```python
from build123d import *

# Parameters (mm, degrees)
BOSS_EXTRUDE1_DEPTH = 25
FILLET1_R           = 5
SKETCH2_R           = 2
CUT_EXTRUDE1_DEPTH  = 5
FILLET2_R           = 5
BOSS_EXTRUDE2_DEPTH = 2.5
FILLET3_R           = 5
FILLET4_R           = 3


with BuildPart() as part:
    # Sketch1 → Boss-Extrude1 (new, symmetric)
    with BuildSketch(Plane(origin=(0, 0, 0), x_dir=(1, 0, 0), z_dir=(0, 1, 0))):
        Polygon((-40, 0), (-20, 0), (-20, 40), (20, 40), (20, 0), (40, 0), (40, 5), (25, 5), (25, 45), (-25, 45), (-25, 5), (-40, 5), align=None)
    extrude(amount=BOSS_EXTRUDE1_DEPTH, both=True)

    # Fillet1
    fillet1_edges = [part.edges().sort_by_distance(p)[0] for p in [
        (-25, 0, -5),
        (-25, 0, -45),
        (25, 0, -45),
        (25, 0, -5),
        (20, 0, -40),
        (-20, 0, -40),
    ]]
    fillet(fillet1_edges, radius=FILLET1_R)

    # Sketch2 → Cut-Extrude1 (cut)
    with BuildSketch(Plane.XY):
        with Locations((-32.5, 20)):
            Circle(SKETCH2_R)
        with Locations((-32.5, -20)):
            Circle(SKETCH2_R)
        with Locations((32.5, -20)):
            Circle(SKETCH2_R)
        with Locations((32.5, 20)):
            Circle(SKETCH2_R)
    extrude(amount=-CUT_EXTRUDE1_DEPTH, mode=Mode.SUBTRACT)

    # Fillet2
    fillet2_edges = [part.edges().sort_by_distance(p)[0] for p in [
        (40, -25, -2.5),
        (-40, -25, -2.5),
        (40, 25, -2.5),
        (-40, 25, -2.5),
    ]]
    fillet(fillet2_edges, radius=FILLET2_R)

    # Sketch3 → Boss-Extrude2 (add, symmetric)
    with BuildSketch(Plane(origin=(0, 0, 0), x_dir=(1, 0, 0), z_dir=(0, 1, 0))):
        Polygon((-40, 5), (-25, 35), (-25, 5), align=None)
    boss_extrude2 = extrude(amount=BOSS_EXTRUDE2_DEPTH, both=True)

    # Mirror5: Boss-Extrude2 across plane
    add(boss_extrude2.mirror(Plane(origin=(0, 0, 0), x_dir=(0, 0, 1), z_dir=(1, 0, 0))))

    # Fillet3
    # the kernel refuses this fillet: 5 mm, written as the material it adds along each edge
    with BuildSketch(Plane(origin=(-30, -2.5, -10), x_dir=(1, 0, 0), z_dir=(0, 0, -1))) as fillet3_piece_1:
        with BuildLine():
            CenterArc((5 - FILLET3_R, FILLET3_R), FILLET3_R, 270, 90)
            Line((5 - FILLET3_R, 0), (5, 0))
            Line((5, 0), (5, FILLET3_R))
        make_face()
    revolve(axis=Axis((-30, -2.5, -10), (0, -1, 0)), revolution_arc=90)
    with BuildSketch(Plane(origin=(-30, 2.5, -10), x_dir=(1, 0, 0), z_dir=(0, 0, -1))) as fillet3_piece_2:
        with BuildLine():
            CenterArc((5 - FILLET3_R, -FILLET3_R), FILLET3_R, 0, 90)
            Line((5 - FILLET3_R, 0), (5, 0))
            Line((5, 0), (5, -FILLET3_R))
        make_face()
    revolve(axis=Axis((-30, 2.5, -10), (0, -1, 0)), revolution_arc=90)
    with BuildSketch(Plane(origin=(-25, -2.5, -47.5), x_dir=(-1, 0, 0), z_dir=(0, 0, 1))) as fillet3_piece_3_section:
        with BuildLine():
            CenterArc((FILLET3_R, FILLET3_R), FILLET3_R, 180, 90)
            Line((0, FILLET3_R), (0, 0))
            Line((0, 0), (FILLET3_R, 0))
        make_face()
    fillet3_piece_3 = extrude(amount=37.5, mode=Mode.PRIVATE)
    fillet3_piece_3 = split(fillet3_piece_3, bisect_by=Plane(origin=(-30.617859864, -3.692357018, -23.764280273), z_dir=(0.894427190999916, 0, 0.44721359549995787)), keep=Keep.TOP, mode=Mode.PRIVATE)
    add(fillet3_piece_3)
    with BuildSketch(Plane(origin=(-25, 2.5, -47.5), x_dir=(0, 1, 0), z_dir=(0, 0, 1))) as fillet3_piece_4_section:
        with BuildLine():
            CenterArc((FILLET3_R, FILLET3_R), FILLET3_R, 180, 90)
            Line((0, FILLET3_R), (0, 0))
            Line((0, 0), (FILLET3_R, 0))
        make_face()
    fillet3_piece_4 = extrude(amount=37.5, mode=Mode.PRIVATE)
    fillet3_piece_4 = split(fillet3_piece_4, bisect_by=Plane(origin=(-30.617859864, 3.692357018, -23.764280273), z_dir=(0.894427190999916, 0, 0.44721359549995787)), keep=Keep.TOP, mode=Mode.PRIVATE)
    add(fillet3_piece_4)
    with BuildSketch(Plane(origin=(-30, 2.5, -5), x_dir=(0, 1, 0), z_dir=(-1, 0, 0))) as fillet3_piece_5_section:
        with BuildLine():
            CenterArc((FILLET3_R, FILLET3_R), FILLET3_R, 180, 90)
            Line((0, FILLET3_R), (0, 0))
            Line((0, 0), (FILLET3_R, 0))
        make_face()
    fillet3_piece_5 = extrude(amount=10, mode=Mode.PRIVATE)
    fillet3_piece_5 = split(fillet3_piece_5, bisect_by=Plane(origin=(-38.518002001, 3.668083757, -7.963995998), z_dir=(0.894427190999916, 0, 0.44721359549995787)), keep=Keep.TOP, mode=Mode.PRIVATE)
    add(fillet3_piece_5)
    with BuildSketch(Plane(origin=(-30, -2.5, -5), x_dir=(0, -1, 0), z_dir=(-1, 0, 0))) as fillet3_piece_6_section:
        with BuildLine():
            CenterArc((FILLET3_R, -FILLET3_R), FILLET3_R, 90, 90)
            Line((0, -FILLET3_R), (0, 0))
            Line((0, 0), (FILLET3_R, 0))
        make_face()
    fillet3_piece_6 = extrude(amount=10, mode=Mode.PRIVATE)
    fillet3_piece_6 = split(fillet3_piece_6, bisect_by=Plane(origin=(-38.518002001, -3.668083757, -7.963995998), z_dir=(0.894427190999916, 0, 0.44721359549995787)), keep=Keep.TOP, mode=Mode.PRIVATE)
    add(fillet3_piece_6)
    with BuildSketch(Plane(origin=(30, -2.5, -10), x_dir=(-1, 0, 0), z_dir=(0, 0, -1))) as fillet3_piece_7:
        with BuildLine():
            CenterArc((5 - FILLET3_R, -FILLET3_R), FILLET3_R, 0, 90)
            Line((5 - FILLET3_R, 0), (5, 0))
            Line((5, 0), (5, -FILLET3_R))
        make_face()
    revolve(axis=Axis((30, -2.5, -10), (0, 1, 0)), revolution_arc=90)
    with BuildSketch(Plane(origin=(30, 2.5, -10), x_dir=(-1, 0, 0), z_dir=(0, 0, -1))) as fillet3_piece_8:
        with BuildLine():
            CenterArc((5 - FILLET3_R, FILLET3_R), FILLET3_R, 270, 90)
            Line((5, FILLET3_R), (5, 0))
            Line((5, 0), (5 - FILLET3_R, 0))
        make_face()
    revolve(axis=Axis((30, 2.5, -10), (0, 1, 0)), revolution_arc=90)
    with BuildSketch(Plane(origin=(25, 2.5, -47.5), x_dir=(0, 1, 0), z_dir=(0, 0, 1))) as fillet3_piece_9_section:
        with BuildLine():
            CenterArc((FILLET3_R, -FILLET3_R), FILLET3_R, 90, 90)
            Line((0, -FILLET3_R), (0, 0))
            Line((0, 0), (FILLET3_R, 0))
        make_face()
    fillet3_piece_9 = extrude(amount=37.5, mode=Mode.PRIVATE)
    fillet3_piece_9 = split(fillet3_piece_9, bisect_by=Plane(origin=(30.617859864, 3.692357018, -23.764280273), z_dir=(-0.894427190999916, 0, 0.44721359549995787)), keep=Keep.TOP, mode=Mode.PRIVATE)
    add(fillet3_piece_9)
    with BuildSketch(Plane(origin=(30, -2.5, -5), x_dir=(0, -1, 0), z_dir=(1, 0, 0))) as fillet3_piece_10_section:
        with BuildLine():
            CenterArc((FILLET3_R, FILLET3_R), FILLET3_R, 180, 90)
            Line((0, FILLET3_R), (0, 0))
            Line((0, 0), (FILLET3_R, 0))
        make_face()
    fillet3_piece_10 = extrude(amount=10, mode=Mode.PRIVATE)
    fillet3_piece_10 = split(fillet3_piece_10, bisect_by=Plane(origin=(38.518002001, -3.668083757, -7.963995998), z_dir=(-0.894427190999916, 0, 0.44721359549995787)), keep=Keep.TOP, mode=Mode.PRIVATE)
    add(fillet3_piece_10)
    with BuildSketch(Plane(origin=(25, -2.5, -47.5), x_dir=(0, -1, 0), z_dir=(0, 0, 1))) as fillet3_piece_11_section:
        with BuildLine():
            CenterArc((FILLET3_R, FILLET3_R), FILLET3_R, 180, 90)
            Line((0, FILLET3_R), (0, 0))
            Line((0, 0), (FILLET3_R, 0))
        make_face()
    fillet3_piece_11 = extrude(amount=37.5, mode=Mode.PRIVATE)
    fillet3_piece_11 = split(fillet3_piece_11, bisect_by=Plane(origin=(30.617859864, -3.692357018, -23.764280273), z_dir=(-0.894427190999916, 0, 0.44721359549995787)), keep=Keep.TOP, mode=Mode.PRIVATE)
    add(fillet3_piece_11)
    with BuildSketch(Plane(origin=(30, 2.5, -5), x_dir=(0, 0, -1), z_dir=(1, 0, 0))) as fillet3_piece_12_section:
        with BuildLine():
            CenterArc((FILLET3_R, FILLET3_R), FILLET3_R, 180, 90)
            Line((0, FILLET3_R), (0, 0))
            Line((0, 0), (FILLET3_R, 0))
        make_face()
    fillet3_piece_12 = extrude(amount=10, mode=Mode.PRIVATE)
    fillet3_piece_12 = split(fillet3_piece_12, bisect_by=Plane(origin=(38.518002001, 3.668083757, -7.963995998), z_dir=(-0.894427190999916, 0, 0.44721359549995787)), keep=Keep.TOP, mode=Mode.PRIVATE)
    add(fillet3_piece_12)

    # Fillet4
    fillet4_edges = [part.edges().sort_by_distance(p)[0] for p in [
        (20, 0, 0),
        (-20, 0, 0),
    ]]
    fillet(fillet4_edges, radius=FILLET4_R)


solid = part.part
```
Could you check a few things on this model? Use its own coordinates, in mm. A direction names the side the tool comes from. Coordinates: 2 decimals unless noted, no trailing zeros. Order: outer loops, then holes, each group sorted by start corner. A loop starts at its lowest first (then second) coordinate and runs counter-clockwise, first axis right, second up. Notation, with made-up numbers: M 24.25,-14.5 L 28.25,-14.5 A11 cw 28.25,-9.5 Z; hole C 7,51.5 d2. An arc over 180 degrees is marked long. Use a Markdown table: item, result. Add a question column.
Q1. If I drill on L1, parallel to Y at x = -32.5, z = -2.95; L2, parallel to X at y = -14.5, z = -28; L3, parallel to Y at x = 32, z = -3, over which ranges is the centre line in solid material (lowest first)?
Q2. I want a section at D-D on z = -22.5. List the corners of the cut face in (x, y) for me, then the cut area to 3 significant figures.
Q3. We'd pull the mould along X, two halves only. Please class faces 6 (the flat face through (-35, -16, -5)), 7 (the cylindrical face through (26.5, -3.93, -19.9)), 8 (the cylindrical face through (19, 0, -38)): pulls with the +X half, pulls with the -X half, needs draft (parallel to the pull), parting line crosses it, or undercut.
Q4. I'm going to push flat-ended pins straight in: pin 1 (2.5 mm diameter, centred on x = -35.5, z = -20, fed in from -Y); pin 2 (6 mm diameter, centred on x = -10.5, y = -17.5, fed in from +Z); pin 3 (2.5 mm diameter, centred on x = 34, z = -18, fed in from +Y); pin 4 (8 mm diameter, centred on x = 36, y = 15.5, fed in from -Z). Where does each tip first touch, or does it pass through?
Q5. I want a section at C-C on y = -4. List the corners of the cut face in (x, z) for me, then the cut area to 3 significant figures.
Q6. I want a section at A-A on z = -14.5. List the corners of the cut face in (x, y) for me.
Q7. I want a section at B-B on x = -32.5. List the corners of the cut face in (y, z) for me, then the cut area to 3 significant figures.
Q8. Which directions (+Z, -Z, +X, -X, +Y, -Y) give clear straight access to the entire face, cutting with the end or side of a thin tool? Please do faces 1 (the cylindrical face through (-20.9, 0.35, -0.86)), 2 (the flat face through (-32, -2.5, -14)), 3 (the cylindrical face through (34.93, 4, -6.43)), 4 (the flat face through (25, 11, -25)), 5 (the flat face through (35, -16, -5)).
Checked values:
| question | item | result |
|---|---|---|
| 1 | L1 | -25 to -22, -18 to 18, 22 to 25 |
| 1 | L2 | -25 to -20, 20 to 25 |
| 1 | L3 | -25 to -21.94, -18.06 to 18.06, 21.94 to 25 |
| 2 | outline | M -31.25,-2.5 L -30,-2.5 A5 cw -25,-7.5 L -25,-25 L -20,-25 L -20,25 L -25,25 L -25,7.5 A5 cw -30,2.5 L -31.25,2.5 Z; M 20,-25 L 25,-25 L 25,-7.5 A5 cw 30,-2.5 L 31.25,-2.5 L 31.25,2.5 L 30,2.5 A5 cw 25,7.5 L 25,25 L 20,25 Z |
| 2 | area | 584 mm² |
| 3 | face 6 | needs draft |
| 3 | face 7 | pulls with the +X half |
| 3 | face 8 | undercut |
| 4 | pin 1 | through |
| 4 | pin 2 | z = -40 |
| 4 | pin 3 | y = 2.5 |
| 4 | pin 4 | z = -5 |
| 5 | outline | M -40,-5 L -39.29,-6.43 L -30,-6.43 A3.57 cw -26.43,-10 L -26.43,-32.14 L -25,-35 L -25,-40 A5 ccw -20,-45 L 20,-45 A5 ccw 25,-40 L 25,-35 L 26.43,-32.14 L 26.43,-10 A3.57 cw 30,-6.43 L 39.29,-6.43 L 40,-5 L 40,0 L 23,0 A3 ccw 20,-3 L 20,-35 A5 cw 15,-40 L -15,-40 A5 cw -20,-35 L -20,-3 A3 ccw -23,0 L -40,0 Z |
| 5 | area | 921 mm² |
| 6 | outline | M -35.25,-2.5 L -30,-2.5 A5 cw -25,-7.5 L -25,-25 L -20,-25 L -20,25 L -25,25 L -25,7.5 A5 cw -30,2.5 L -35.25,2.5 Z; M 20,-25 L 25,-25 L 25,-7.5 A5 cw 30,-2.5 L 35.25,-2.5 L 35.25,2.5 L 30,2.5 A5 cw 25,7.5 L 25,25 L 20,25 Z |
| 7 | outline | M -25,-5 L -22,-5 L -22,0 L -25,0 Z; M -18,-5 L -7.5,-5 A5 cw -2.5,-10 L -2.5,-20 L 2.5,-20 L 2.5,-10 A5 cw 7.5,-5 L 18,-5 L 18,0 L -18,0 Z; M 22,-5 L 25,-5 L 25,0 L 22,0 Z |
| 7 | area | 296 mm² |
| 8 | face 1 | +Z, +Y, -Y |
| 8 | face 2 | -Z, -X, -Y |
| 8 | face 3 | -Z, +X, +Y |
| 8 | face 4 | -Z, +X |
| 8 | face 5 | -Z, +X, -Y |
